from build123d import *

# Parameters (mm, degrees)
SKETCH1_R           = 2
BOSS_EXTRUDE1_DEPTH = 83.5


with BuildPart() as part:
    # Sketch1 → Boss-Extrude1 (new, symmetric)
    with BuildSketch(Plane.XY):
        Polygon((10, 4.610379336), (10, 10), (4.610379336, 10), (3.1, 10), (3.1, 8.5), (5.5, 8.5), (5.5, 6.860660172), (2.839339828, 3.9), (0.519615242, 3.9), (-0.519615242, 3.9), (-2.839339828, 3.9), (-5.5, 6.860660172), (-5.5, 8.5), (-3.1, 8.5), (-3.1, 10), (-4.610379336, 10), (-10, 10), (-10, 4.610379336), (-10, 3.1), (-8.5, 3.1), (-8.5, 5.5), (-6.860660172, 5.5), (-3.9, 2.839339828), (-3.9, 0.519615242), (-3.9, -0.519615242), (-3.9, -2.839339828), (-6.860660172, -5.5), (-8.5, -5.5), (-8.5, -3.1), (-10, -3.1), (-10, -4.610379336), (-10, -10), (-4.610379336, -10), (-3.1, -10), (-3.1, -8.5), (-5.5, -8.5), (-5.5, -6.860660172), (-2.839339828, -3.9), (-0.519615242, -3.9), (0.519615242, -3.9), (2.839339828, -3.9), (5.5, -6.860660172), (5.5, -8.5), (3.1, -8.5), (3.1, -10), (4.610379336, -10), (10, -10), (10, -4.610379336), (10, -3.1), (8.5, -3.1), (8.5, -5.5), (6.860660172, -5.5), (3.9, -2.839339828), (3.9, -0.519615242), (3.9, 0.519615242), (3.9, 2.839339828), (6.860660172, 5.5), (8.5, 5.5), (8.5, 3.1), (10, 3.1), align=None)
        with Locations(Location((0, 0, 0), (0, 0, 180))):
            Circle(SKETCH1_R, mode=Mode.SUBTRACT)
    extrude(amount=BOSS_EXTRUDE1_DEPTH, both=True)


solid = part.part
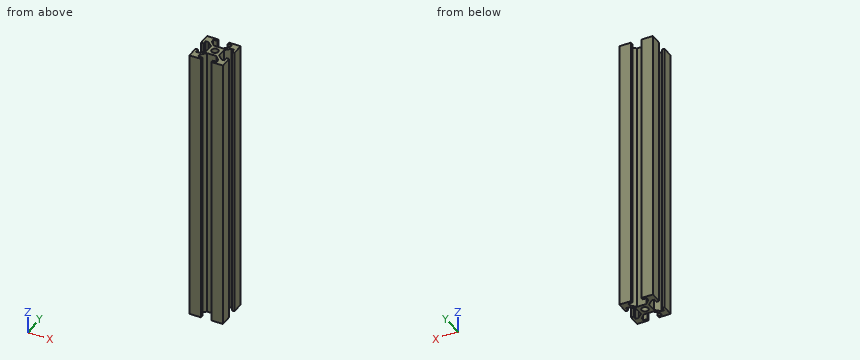
Can you work these out from the model? Positions are in its coordinate system, mm. Give positions to 0.01 mm unless a question says otherwise; leave off trailing zeros. Loops run counter-clockwise (first coordinate to the right, second up) from the corner with the lowest first, then second, coordinate; pieces in that order, holes last. Notation, with made-up numbers: M 31.25,53 L 86.25,53 A5 cw 86.25,57 Z; hole C -35,56 d4. An arc over 180 degrees is marked long. One line per item, written item: value. Start each with the question number.
1) If I drill on line 1 (Y direction, x = 0, z = -43.5); line 2 (X direction, y = -9, z = -57.5); line 3 (X direction, y = 8, z = -67), over which ranges is the centre line in solid material (lowest first)? Write a range as [from, to].
2) I'm going to push a flat-ended pin straight in: pin 1 (1.7 mm diameter, centred on x = -1, z = 11.5, fed in from -Y). Where does the tip first touch, or does it pass through?
3) If we section it at A-A, the plane y = 0: Write out the boundary of the cut face in (x, z), and give its area (3 significant figures).
Completed:
1. line 1: y = [-3.9, -2], [2, 3.9]
1. line 2: x = [-10, -3.1], [3.1, 10]
1. line 3: x = [-10, -5.5], [5.5, 10]
2. pin 1: stops at y = -3.9
3. outline: M -3.9,-83.5 L -2,-83.5 L -2,83.5 L -3.9,83.5 Z; M 2,-83.5 L 3.9,-83.5 L 3.9,83.5 L 2,83.5 Z
3. area: 635 mm^2
